Could you check a few things on this drawing? It's one solid part, dimensions in mm from its lowest x, y, z. A direction names the side the tool comes from. Give positions to 0.01 mm unless a question says otherwise; leave off trailing zeros. Loops run counter-clockwise (first coordinate to the right, second up) from the corner with the lowest first, then second, coordinate; pieces in that order, holes last. Notation, with made-up numbers: (3, 85) -> (31, 85) arc R15 cw to (31, 98) -> close; hole circle Ø9 at (34.25, -39.5). An arc over 180 degrees is marked (long way). Use CSV: the item, a comma, the result in double quotes.
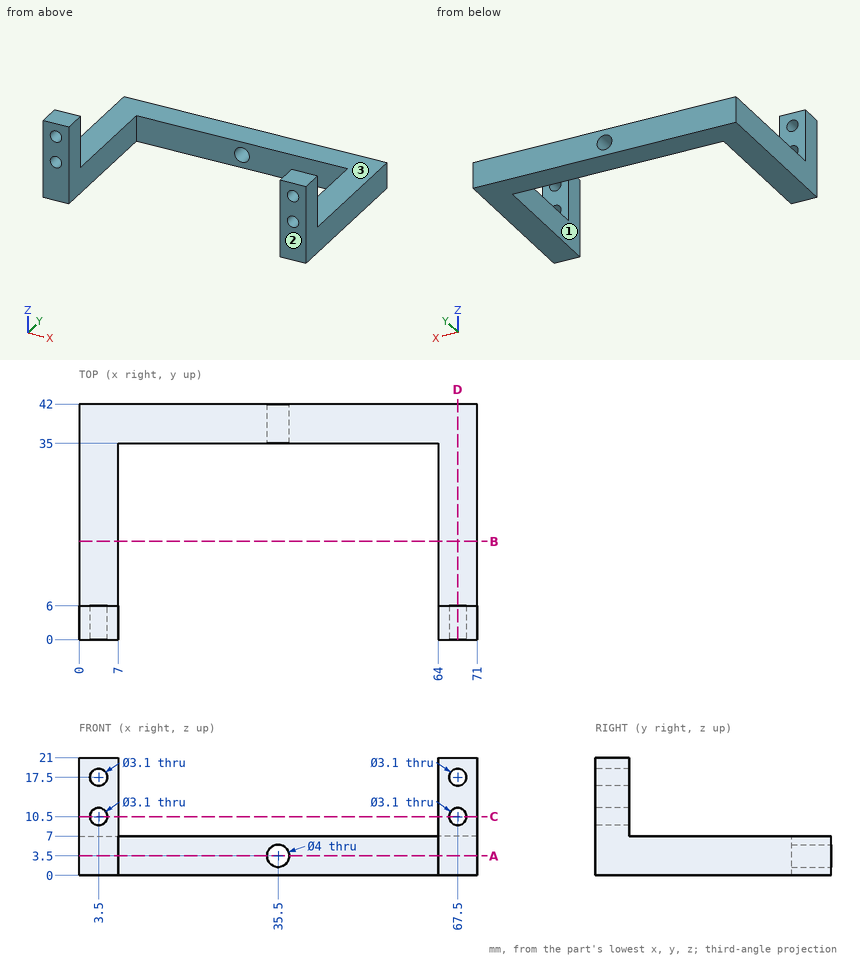
(1) If we section it at A-A, the plane z = 3.5: Write out the boundary of the cut face in (x, y), then the cut area to 3 significant figures.
Answer sheet:
outline,"(0, 0) -> (7, 0) -> (7, 35) -> (33.5, 35) -> (33.5, 42) -> (0, 42) -> close; (37.5, 35) -> (64, 35) -> (64, 0) -> (71, 0) -> (71, 42) -> (37.5, 42) -> close"
area,"959 mm2"
(2) If I drill on L1, parallel to Z at x = 3.5, y = 4.7; L2, parallel to X at y = 4.1, z = 10.5; L3, parallel to X at y = 5.5, z = 1, over which ranges is the centre line in solid material (lowest first)? Write a range as from..to.
Answer sheet:
L1,"z = 0..8.95, 12.05..15.95, 19.05..21"
L2,"x = 0..1.95, 5.05..7, 64..65.95, 69.05..71"
L3,"x = 0..7, 64..71"
(3) If we section it at C-C, the plane z = 10.5: Write out the boundary of the cut face in (x, y).
Answer sheet:
outline,"(0, 0) -> (1.95, 0) -> (1.95, 6) -> (0, 6) -> close; (5.05, 0) -> (7, 0) -> (7, 6) -> (5.05, 6) -> close; (64, 0) -> (65.95, 0) -> (65.95, 6) -> (64, 6) -> close; (69.05, 0) -> (71, 0) -> (71, 6) -> (69.05, 6) -> close"
(4) If we section it at B-B, the plane y = 17.5: Write out the boundary of the cut face in (x, z).
Answer sheet:
outline,"(0, 0) -> (7, 0) -> (7, 7) -> (0, 7) -> close; (64, 0) -> (71, 0) -> (71, 7) -> (64, 7) -> close"
(5) Will these pins go through, and if not, where does the flat tip stop? pin 1 Ø5.5 at (x, z) = (66.5, 15.5) entering from +Y; pin 2 Ø2 at (x, z) = (34.5, 3) entering from -Y.
Answer sheet:
pin 1,"stops at y = 6"
pin 2,"stops at y = 35"
(6) If we section it at D-D, the plane x = 67.5: Write out the boundary of the cut face in (y, z).
Answer sheet:
outline,"(0, 0) -> (42, 0) -> (42, 7) -> (6, 7) -> (6, 8.95) -> (0, 8.95) -> close; (0, 12.05) -> (6, 12.05) -> (6, 15.95) -> (0, 15.95) -> close; (0, 19.05) -> (6, 19.05) -> (6, 21) -> (0, 21) -> close"
(7) Which directions (+Z, -Z, +X, -X, +Y, -Y) give clear straight access to the entire face, cutting with the end or side of a thin tool? Please do the marked faces 1, 2 and 3.
Answer sheet:
face 1,"+Z, -Z, -Y"
face 2,"+Z, -Z, +X, -X, -Y"
face 3,"+Z, +X, -X, +Y"
